Design review of the part shown in the three views and the two pictorial views. Dimensions are in mm from the part's minimum x, y and z. A direction names the side the tool comes from. Coordinates: 2 decimals unless noted, no trailing zeros. Write each loop counter-clockwise with the first axis right and the second up, starting at its lowest first coordinate (ties: lowest second). Pieces come first, ordered by that corner, then holes. Notation, with made-up numbers: (73.25, 22.25) -> (83.25, 22.25) arc R20 ccw to (83.25, 54.25) -> close; hole circle Ø2 at (31.25, 27). An arc over 180 degrees is marked (long way). Write each question's results on one line, items separated by ' | '.
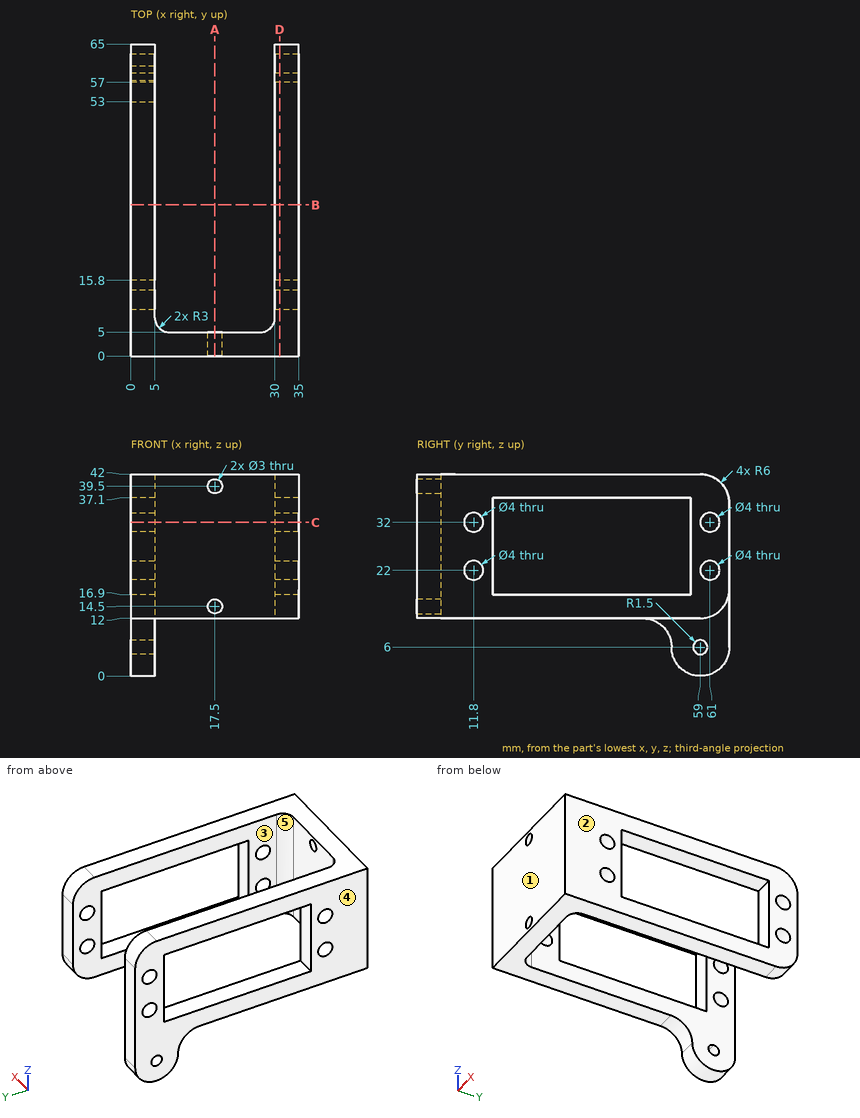
Q1. Add section D-D (x = 31). Write out the cut boundary in (y, z).
Solution:
outline: (0, 12) -> (59, 12) arc R6 ccw to (65, 18) -> (65, 36) arc R6 ccw to (59, 42) -> (0, 42) -> close; hole circle Ø4 at (11.8, 22); hole circle Ø4 at (11.8, 32); hole (15.8, 16.9) -> (57, 16.9) -> (57, 37.1) -> (15.8, 37.1) -> close; hole circle Ø4 at (61, 22); hole circle Ø4 at (61, 32)
Q2. Draft analysis for pull direction X (two halves, no side actions). For the marked faces 1, 2 and 3, state which applies: pulls with the +X half, pulls with the -X half, needs draft (parallel to the pull), parting line crosses it, or undercut.
Solution:
face 1: needs draft | face 2: pulls with the +X half | face 3: undercut
Q3. Add section B-B (y = 31.5). Write out the cut boundary in (x, z).
Solution:
outline: (0, 12) -> (5, 12) -> (5, 16.9) -> (0, 16.9) -> close; (0, 37.1) -> (5, 37.1) -> (5, 42) -> (0, 42) -> close; (30, 12) -> (35, 12) -> (35, 16.9) -> (30, 16.9) -> close; (30, 37.1) -> (35, 37.1) -> (35, 42) -> (30, 42) -> close
Q4. Machinability: for the marked faces 4 and 5, which of the approach directions +Z, -Z, +X, -X, +Y, -Y give a long, thin tool a straight path to every point of the face, cutting with its end or side? Answer none if there is none.
Solution:
face 4: +Z, -Z, -X, +Y, -Y | face 5: +Z, -Z, +Y
Q5. Add section A-A (x = 17.5). Write out the cut boundary in (y, z).
Solution:
outline: (0, 12) -> (5, 12) -> (5, 13) -> (0, 13) -> close; (0, 16) -> (5, 16) -> (5, 38) -> (0, 38) -> close; (0, 41) -> (5, 41) -> (5, 42) -> (0, 42) -> close
Q6. Clearance check with flat-ended pins moving along their axes: P1, Ø5, axis at y = 61, z = 22, coming from the +X side; P2, Ø12, axis at x = 27.5, y = 17, coming from the -Z side; P3, Ø3.5, axis at x = 17.5, z = 14.5, coming from the +Y side. State where each tip first meets the part, or that it passes through.
Solution:
P1: x = 35 | P2: z = 12 | P3: y = 5
Q7. Add section C-C (z = 32). Count the separate pieces of the cut face and the enclosed holes in it, plus the area to 3 significant figures.
Solution:
separate pieces: 7 | enclosed holes: 0 | area: 287 mm²
Q8. For line 1 (Y direction, x = 3, z = 22); line 2 (Y direction, x = 2, z = 6); line 3 (X direction, y = 49, z = 39.5), list the stretches that pass through material, from the lowest coordinate up. Write a range as from..to.
Solution:
line 1: 0..9.8, 13.8..15.8, 57..59, 63..65 | line 2: 53..57.5, 60.5..65 | line 3: 0..5, 30..35
